```python
from build123d import *

# Parameters (mm, degrees)
SKETCH_1_W                      = 186
SKETCH_1_H                      = 149
FLOOR_T3_DEPTH                  = 3
SKETCH_2_W                      = 186
SKETCH_2_H                      = 149
SKETCH_2_W_2                    = 180
SKETCH_2_H_2                    = 143
WALLS_T3_DEPTH80_DEPTH          = 83
SKETCH_3_W                      = 11
SKETCH_3_H                      = 8
SERVO_STAND_RELIEF_W8_H58_DEPTH = 58
SKETCH_4_W                      = 11
SKETCH_4_H                      = 17
SERVO_EARS_RELIEF_V3_DEPTH      = 58


with BuildPart() as part:
    # 草图1 → Floor_T3 (new body)
    with BuildSketch(Plane.XY):
        with Locations((93, 74.5)):
            Rectangle(SKETCH_1_W, SKETCH_1_H)
    extrude(amount=FLOOR_T3_DEPTH)

    # 草图2 → Walls_T3_depth80 (add)
    with BuildSketch(Plane.XY):
        with Locations((93, 74.5)):
            Rectangle(SKETCH_2_W, SKETCH_2_H)
        with Locations((93, 74.5)):
            Rectangle(SKETCH_2_W_2, SKETCH_2_H_2, mode=Mode.SUBTRACT)
    extrude(amount=WALLS_T3_DEPTH80_DEPTH)

    # 草图3 → Servo_stand_relief_W8_H58 (cut)
    with BuildSketch(Plane.XY):
        with Locations((4.5, 23.5)):
            Rectangle(SKETCH_3_W, SKETCH_3_H)
    extrude(amount=SERVO_STAND_RELIEF_W8_H58_DEPTH, mode=Mode.SUBTRACT)

    # 草图4 → Servo_ears_relief_v3 (cut)
    with BuildSketch(Plane.XY):
        with Locations((4.5, 19)):
            Rectangle(SKETCH_4_W, SKETCH_4_H)
    extrude(amount=SERVO_EARS_RELIEF_V3_DEPTH, mode=Mode.SUBTRACT)


solid = part.part
```
Could you check a few things on this model? Use its own coordinates, in mm. A direction names the side the tool comes from. Give positions to 0.01 mm unless a question says otherwise; leave off trailing zeros. Order: outer loops, then holes, each group sorted by start corner. A loop starts at its lowest first (then second) coordinate and runs counter-clockwise, first axis right, second up.
Q1. If I drill on line 1 along Y through (x, z) = (47.5, 39.5); line 2 along X through (y, z) = (115.5, 45); line 3 along Z through (x, y) = (38, 39), over which ranges is the centre line in solid material (lowest first)?
Q2. I'm going to push flat-ended pins straight in: P1, Ø3, axis at x = 114, y = 85, coming from the +Z side; P2, Ø11, axis at x = 7, z = 20.5, coming from the -Y side; P3, Ø3.5, axis at x = 1, y = 23, coming from the -Z side; P4, Ø1.5, axis at y = 22.5, z = 1, coming from the -X side. Where does each tip first touch, or does it pass through?
Q3. Suppose I cut it at B-B, the plane y = 46. Write out the boundary of the cut face in (x, z), and give its area (3 significant figures).
Q4. For faces 1 (the flat face through (2.7, 27.5, 22.1)), 2 (the flat face through (93, 147, 83)), 3 (the flat face through (92, 3, 42)), which set-ups out of +Z, -Z, +X, -X, +Y, -Y let a thin tool reach every point of the face, with its end or its side?
Q5. Suppose I cut it at A-A, the plane z = 75. Write out the boundary of the cut face in (x, y).
Q6. Suppose I cut it at C-C, the plane x = 40. Write out the boundary of the cut face in (y, z).
Q7. Suppose I cut it at D-D, the plane z = 35. Write out the boundary of the cut face in (x, y).
Q8. We'd pull the mould along Y, two halves only. Please class faces 4 (the flat face through (3, 73, 42)), 5 (the flat face through (92, 149, 41)), 6 (the flat face through (186, 73, 41)), 7 (the flat face through (92, 0, 41)): +Y half, -Y half, draft (parallel to the pull), parting line (faces both ways), or undercut.
Solution:
1. line 1: y = 0 to 3, 146 to 149
1. line 2: x = 0 to 3, 183 to 186
1. line 3: z = 0 to 3
2. P1: stops at z = 3
2. P2: stops at y = 0
2. P3: stops at z = 58
2. P4: stops at x = 10
3. outline: (0, 0) - (186, 0) - (186, 83) - (183, 83) - (183, 3) - (3, 3) - (3, 83) - (0, 83) - close
3. area: 1,040 mm2
4. face 1: -Z, -X
4. face 2: +Z, +X, -X, +Y, -Y
4. face 3: +Z
5. outline: (0, 0) - (186, 0) - (186, 149) - (0, 149) - close; hole (3, 3) - (183, 3) - (183, 146) - (3, 146) - close
6. outline: (0, 0) - (149, 0) - (149, 83) - (146, 83) - (146, 3) - (3, 3) - (3, 83) - (0, 83) - close
7. outline: (0, 0) - (186, 0) - (186, 149) - (0, 149) - (0, 27.5) - (3, 27.5) - (3, 146) - (183, 146) - (183, 3) - (3, 3) - (3, 10.5) - (0, 10.5) - close
8. face 4: undercut
8. face 5: +Y half
8. face 6: draft
8. face 7: -Y half
